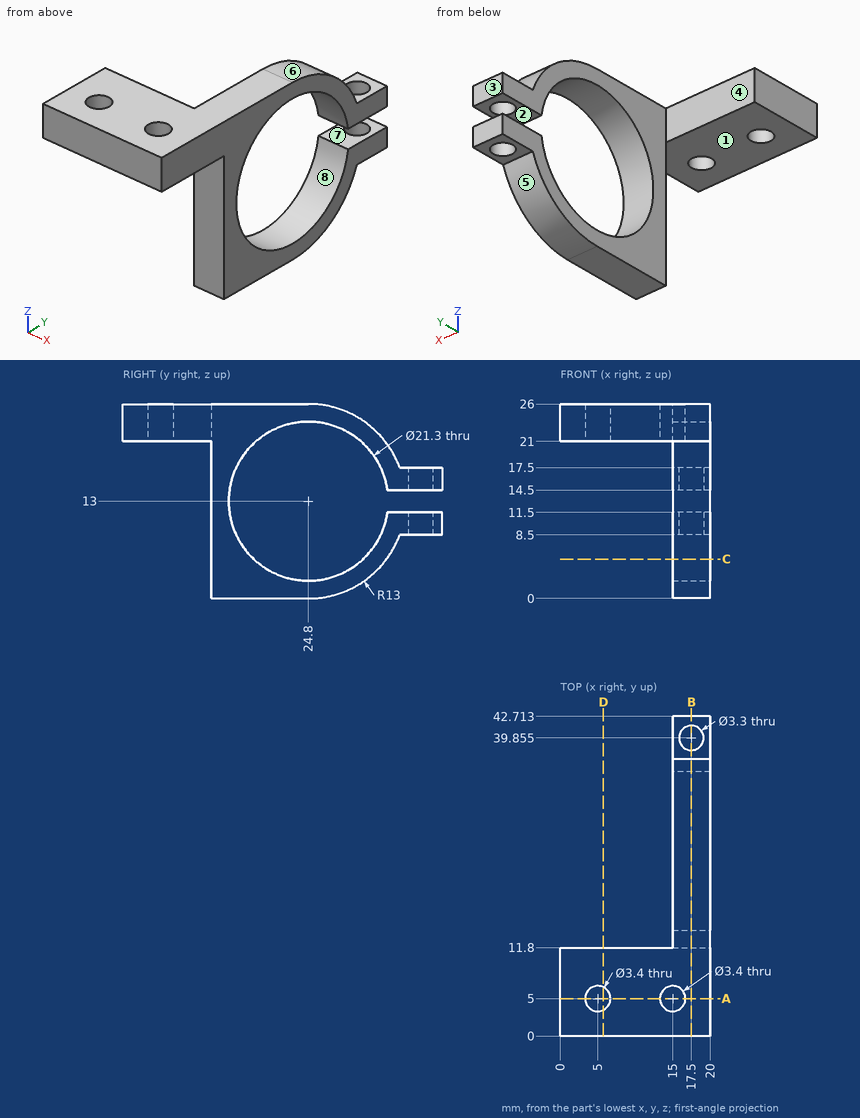
Here's the drawing with two shaded views (mm, measured from the low corner). I have some questions. A direction names the side the tool comes from. Give positions to 0.01 mm unless a question says otherwise; leave off trailing zeros. Loops run counter-clockwise (first coordinate to the right, second up) from the corner with the lowest first, then second, coordinate; pieces in that order, holes last. Notation, with made-up numbers: M 60,28 L 71,28 A31 ccw 71,63 Z; hole C -17.5,38.5 d1. An arc over 180 degrees is marked long. Use one line per item in the form item = value. Start each with the question number.
(1) I want a section at C-C, the plane z = 5.25. Write out the boundary of the cut face in (x, y) (1 decimal).
(2) I want a section at A-A, the plane y = 5. Write out the boundary of the cut face in (x, z), and give its area (3 significant figures).
(3) On a 3-axis mill with a long thin cutter (end or side, diameter ignored), from which of +Z, -Z, +X, -X, +Y, -Y can I reach the whole of each face in a straight line? I mean the marked faces 1, 2, 3, 4 and 5. Say none if no direction works.
(4) Please list where these lines run through material, in increasing order: line 1 (Y direction, x = 5, z = 24.65); line 2 (Y direction, x = 15.5, z = 22.25) (1 decimal); line 3 (X direction, y = 12, z = 20).
(5) I want a section at D-D, the plane x = 5.75. Write out the boundary of the cut face in (y, z).
(6) I'm going to push flat-ended pins straight in: P1, Ø4.5, axis at x = 15, y = 5, coming from the -Z side; P2, Ø10, axis at y = 31.5, z = 19, coming from the -X side; P3, Ø5.5, axis at x = 6.5, z = 22.5, coming from the +Y side. Where does each tip first touch, or does it pass through?
(7) I want a section at B-B, the plane x = 17.5. State how many separate pieces and enclosed holes the cut face has, and give its area (3 significant figures).
(8) Thinking about a two-plate mould opening in Y: for the marked faces 6, 7 and 8, which applies, released by +Y, released by -Y, zero draft, split by the parting line, or undercut?
Worked out:
q1.outline = M 15,11.8 L 20,11.8 L 20,17.5 L 15,17.5 Z; M 15,32.1 L 20,32.1 L 20,35.2 L 15,35.2 Z
q2.outline = M 0,21 L 3.3,21 L 3.3,26 L 0,26 Z; M 6.7,21 L 13.3,21 L 13.3,26 L 6.7,26 Z; M 16.7,21 L 20,21 L 20,26 L 16.7,26 Z
q2.area = 66.0 mm²
q3.face_1 = -Z, +X, -X, -Y
q3.face_2 = +X, -X, +Y
q3.face_3 = +Z, -Z, +X, -X, +Y
q3.face_4 = +Z, -Z, -X, +Y
q3.face_5 = -Z, +X, -X, +Y
q4.line_1 = 0 to 3.3, 6.7 to 11.8
q4.line_2 = 0 to 3.4, 6.6 to 19.5, 30.1 to 33.9
q4.line_3 = 15 to 20
q5.outline = M 0,21 L 3.47,21 L 3.47,26 L 0,26 Z; M 6.53,21 L 11.8,21 L 11.8,26 L 6.53,26 Z
q6.P1 = 21
q6.P2 = 15
q6.P3 = 11.8
q7.separate_pieces = 3
q7.enclosed_holes = 0
q7.area = 311 mm²
q8.face_6 = released by +Y
q8.face_7 = zero draft
q8.face_8 = undercut
